```python
from build123d import *

# Parameters (mm, degrees)
F1_DEPTH = 25
F2_R     = 24.99999
F3_R     = 24.99999
F4_R     = 24.99999
F5_R     = 24.99999


# Not quite as in the source:
# - a fillet or chamfer is up to 0.001 mm smaller than in the source, because OpenCascade refuses the exact size


with BuildPart() as f1:
    # F0 (on Front) → F1 (new body)
    with BuildSketch(Plane.XZ):
        with BuildLine():
            ThreePointArc((55.4895948443, 54.5060273456), (16.4576480368, 38.7445048189), (0.0021987788, 0))
            Line((0.0021987788, 0), (177, 0))
            Line((177, 0), (177, 25))
            Line((177, 25), (377, 25))
            Line((377, 25), (377, 0))
            Line((377, 0), (554, 0))
            Line((554, 0), (554, 25))
            Line((554, 25), (754, 25))
            Line((754, 25), (754, 0))
            Line((754, 0), (931, 0))
            Line((931, 0), (931, 25))
            Line((931, 25), (1131, 25))
            Line((1131, 25), (1131, 0))
            Line((1131, 0), (1308, 0))
            Line((1308, 0), (1308, 25))
            Line((1308, 25), (1508, 25))
            Line((1508, 25), (1508, 0))
            Line((1508, 0), (1685, 0))
            ThreePointArc((1685, 0), (1642.0718401331, 29.7373237733), (1591.0429702736, 40.8364127275))
            Line((1591.0429702736, 40.8364127275), (55.4895948443, 54.5060273456))
        make_face()
    extrude(amount=F1_DEPTH)

    # F2 (radius 25 in the source; OpenCascade refuses exactly that, so slightly less here)
    f2_edges = [f1.edges().sort_by_distance(p)[0] for p in [
        (177, -12.5, 25),
    ]]
    fillet(f2_edges, radius=F2_R)

    # F3 (radius 25 in the source; OpenCascade refuses exactly that, so slightly less here)
    f3_edges = [f1.edges().sort_by_distance(p)[0] for p in [
        (377, -12.5, 25),
    ]]
    fillet(f3_edges, radius=F3_R)

    # F4 (radius 25 in the source; OpenCascade refuses exactly that, so slightly less here)
    f4_edges = [f1.edges().sort_by_distance(p)[0] for p in [
        (754, -12.5, 25),
        (1131, -12.5, 25),
    ]]
    fillet(f4_edges, radius=F4_R)

    # F5 (radius 25 in the source; OpenCascade refuses exactly that, so slightly less here)
    f5_edges = [f1.edges().sort_by_distance(p)[0] for p in [
        (1508, -12.5, 25),
        (554, -12.5, 25),
        (931, -12.5, 25),
        (1308, -12.5, 25),
    ]]
    fillet(f5_edges, radius=F5_R)


solid = f1.part
```
Part model, mm, in its own coordinate system. Round coordinates to 2 decimals unless told otherwise and drop trailing zeros. Loops run counter-clockwise (first coordinate to the right, second up) from the corner with the lowest first, then second, coordinate; pieces in that order, holes last. Notation, with made-up numbers: (83.5, 6.5) -> (139.5, 6.5) arc R21 ccw to (139.5, 39.5) -> close; hole circle Ø6 at (-37.5, 79.25). An arc over 180 degrees is marked (long way). Use CSV: the item, a comma, the result in double quotes. Start each with the question number.
1) Wall check: L1, parallel to X at y = -9.5, z = 23; L2, parallel to X at y = -18, z = 5; L3, parallel to Z at x = 88, y = -20.75. Give the ranges that are in metal, low to high. Write a range as [from, to].
2) Cut at B-B, the plane z = 10. Write the cut outline in (x, y), plus the area to 3 significant figures.
3) Cut at D-D, the plane x = 281. Write the cut outline in (y, z), plus the area to 3 significant figures.
4) Drop flat-ended pins along their axis: P1, Ø1.5, axis at x = 928, y = -6.5, coming from the -Z side; P2, Ø1, axis at y = -9.5, z = 24, coming from the +X side; P3, Ø6, axis at x = 671, y = -4, coming from the -Z side; P4, Ø6, axis at y = -12.5, z = 23.5, coming from the +X side. Give the stop position or say it passes through.
5) Cut at C-C, the plane x = 782. Write the cut outline in (y, z), plus the area to 3 significant figures.
Determined:
1,L1,"x = [5.27, 192.2], [361.8, 569.2], [738.8, 946.2], [1115.8, 1323.2], [1492.8, 1655.47]"
1,L2,"x = [0.27, 177.51], [376.49, 554.51], [753.49, 931.51], [1130.49, 1308.51], [1507.49, 1679.9]"
1,L3,"z = [0, 54.22]"
2,outline,"(1.01, -25) -> (179.09, -25) -> (179.09, 0) -> (1.01, 0) -> close; (374.91, -25) -> (556.09, -25) -> (556.09, 0) -> (374.91, 0) -> close; (751.91, -25) -> (933.09, -25) -> (933.09, 0) -> (751.91, 0) -> close; (1128.91, -25) -> (1310.09, -25) -> (1310.09, 0) -> (1128.91, 0) -> close; (1505.91, -25) -> (1674.2, -25) -> (1674.2, 0) -> (1505.91, 0) -> close"
2,area,"22,200 mm2"
3,outline,"(-25, 25) -> (0, 25) -> (0, 52.5) -> (-25, 52.5) -> close"
3,area,"687 mm2"
4,P1,"stops at z = 0"
4,P2,"stops at x = 1654.59"
4,P3,"stops at z = 25"
4,P4,"stops at x = 1659.64"
5,outline,"(-25, 0) -> (0, 0) -> (0, 48.04) -> (-25, 48.04) -> close"
5,area,"1,200 mm2"
